Check sheet for the modelled part. Datum: model origin and axes. Units: mm. Round coordinates to 2 decimals unless told otherwise and drop trailing zeros. Write each loop counter-clockwise with the first axis right and the second up, starting at its lowest first coordinate (ties: lowest second). Pieces come first, ordered by that corner, then holes. Notation, with made-up numbers: (-20, 10.5) -> (-12, 10.5) arc R16 ccw to (-12, 36.5) -> close; hole circle Ø11 at (24.5, -38.75). An arc over 180 degrees is marked (long way). Put each result on its own line as item: value. Start each with the question number.
from build123d import *

# Parameters (mm, degrees)
EXTRUSION1_DEPTH                               = 300
FRAISAGE_POUR_VIS_T_TE_FRAIS_E_M41_D           = 4.5
FRAISAGE_POUR_VIS_T_TE_FRAIS_E_M41_CSINK_D     = 5.5
FRAISAGE_POUR_VIS_T_TE_FRAIS_E_M41_CSINK_ANGLE = 90


with BuildPart() as part:
    # Esquisse1 → Extrusion1 (new body)
    with BuildSketch(Plane.XY):
        with BuildLine():
            Line((-38.885451278, -19.821642953), (-4.885451278, -19.821642953))
            Line((-4.885451278, -19.821642953), (-4.885451278, -15.321642953))
            Line((-4.885451278, -15.321642953), (-14.885451278, -15.321642953))
            Line((-14.885451278, -15.321642953), (-14.885451278, -11.321642953))
            Line((-14.885451278, -11.321642953), (-18.885451278, -4.821642953))
            ThreePointArc((-18.885451278, -4.821642953), (-21.78726352, 6.400322803), (-24.885451278, -4.769021956))
            Line((-24.885451278, -4.769021956), (-28.885451278, -11.321642953))
            Line((-28.885451278, -11.321642953), (-28.885451278, -15.321642953))
            Line((-28.885451278, -15.321642953), (-38.885451278, -15.321642953))
            Line((-38.885451278, -15.321642953), (-38.885451278, -19.821642953))
        make_face()
    extrude(amount=EXTRUSION1_DEPTH)

    # Fraisage pour vis à tête fraisée M41 (through all)
    with Locations(Plane(origin=(-33.885451278, -15.321642953, 50), x_dir=(1, 0, 0), z_dir=(0, 1, 0))):
        with Locations((0, 0), (0, -100), (0, -200), (24, -200), (24, -100), (24, 0)):
            CounterSinkHole(FRAISAGE_POUR_VIS_T_TE_FRAIS_E_M41_D / 2, FRAISAGE_POUR_VIS_T_TE_FRAIS_E_M41_CSINK_D / 2, counter_sink_angle=FRAISAGE_POUR_VIS_T_TE_FRAIS_E_M41_CSINK_ANGLE)


solid = part.part
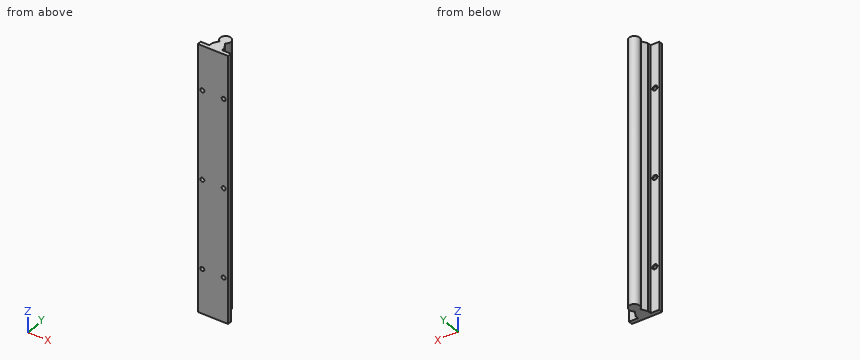
1. Gauge pin test, flat ends, axial feed: P1, Ø2, axis at y = -12.5, z = 207, coming from the -X side; P2, Ø5, axis at x = -33.89, z = 150, coming from the +Y side; P3, Ø1.2, axis at y = -13, z = 99.5, coming from the +X side. Record the tip position at first contact, or that the pin passes through.
2. Section check B-B, the plane y = -1.25. Enter the section's corners in (x, z), then the cut area to 3 significant figures.
3. Section check A-A, the plane z = 99. Enter the section's corners in (x, y), then the cut area to 3 significant figures.
4. Material ranges on L1, parallel to X at y = -17.9, z = 50; L2, parallel to Y at x = -13, z = 199; L3, parallel to Z at x = -9, y = -18, recorded low to high. Write a range as [from, to].
Reply:
1. P1: stops at x = -28.89
1. P2: stops at y = -15.57
1. P3: stops at x = -14.89
2. outline: (-27.61, 0) -> (-16.07, 0) -> (-16.07, 300) -> (-27.61, 300) -> close
2. area: 3,460 mm2
3. outline: (-38.89, -19.82) -> (-4.89, -19.82) -> (-4.89, -15.32) -> (-14.89, -15.32) -> (-14.89, -11.32) -> (-18.89, -4.82) arc R6 ccw (long way) to (-24.89, -4.77) -> (-28.89, -11.32) -> (-28.89, -15.32) -> (-38.89, -15.32) -> close
3. area: 384 mm2
4. L1: x = [-38.89, -36.14], [-31.64, -12.14], [-7.64, -4.89]
4. L2: y = [-19.82, -15.32]
4. L3: z = [0, 47.93], [52.07, 147.93], [152.07, 247.93], [252.07, 300]
